```python
from build123d import *

# Parameters (mm, degrees)
F1_DEPTH = 10
F2_R     = 2


# Not quite as in the source:
# - ends of sketch curves that miss each other by under 0.0002 mm in the source are joined


with BuildPart() as f1:
    # F0 (on Front) → F1 (new body)
    with BuildSketch(Plane.XZ):
        Polygon((-0.0010415313, 0.600002712), (-2.25, 0.6039066758), (-2.25, 10), (-5.25, 10), (-5.25, 3), (-10, 3), (-10, 0), (0, 0), align=None)
        Polygon((0.0010415376, 0.599999096), (-0.0010415313, 0.600002712), (0, 0), align=None)
        Polygon((2.25, 0.6039066758), (0.0010415313, 0.600002712), (0, 0), (10, 0), (10, 3), (5.25, 3), (5.25, 10), (2.25, 10), align=None)
    extrude(amount=F1_DEPTH)

    # F2
    f2_edges = [f1.edges().sort_by_distance(p)[0] for p in [
        (-5.25, -5, 3),
        (5.25, -5, 3),
        (10, -5, 3),
        (5.25, -5, 10),
        (-5.25, -5, 10),
        (-10, -5, 3),
        (-10, -10, 1.5),
        (-10, 0, 1.5),
        (10, -10, 1.5),
        (10, 0, 1.5),
    ]]
    fillet(f2_edges, radius=F2_R)


solid = f1.part
```
Part model, mm, in its own coordinate system. A direction names the side the tool comes from. Round coordinates to 2 decimals unless told otherwise and drop trailing zeros. Write each loop counter-clockwise with the first axis right and the second up, starting at its lowest first coordinate (ties: lowest second). Pieces come first, ordered by that corner, then holes. Notation, with made-up numbers: M 40.25,-27 L 81.25,-27 A36 ccw 81.25,11 Z; hole C 39,18.25 d4. An arc over 180 degrees is marked long. One line per question, with ' | ' between items.
(1) Pin check, flat tips, straight feed: pin 1 (0.6 mm diameter, centred on x = 8, y = -3.5, fed in from +Z); pin 2 (2.5 mm diameter, centred on y = -2.5, z = 6.5, fed in from +X); pin 3 (2.5 mm diameter, centred on y = -4.5, z = 7, fed in from -X). Stop position of each tip, or through.
Answer key:
pin 1: stops at z = 3 | pin 2: stops at x = 5.25 | pin 3: stops at x = -5.25
(2) Saw through at D-D on x = -7.5. Write the cut outline in (y, z).
Answer key:
outline: M -10,0 L 0,0 L 0,3 L -10,3 Z
(3) 3-axis set-ups, long thin cutter, end or side, ignore diameter. For faces 1 (the face through (5.85, -5.07, 3.57)), 2 (the face through (2.25, -5, 5)): which of +Z, -Z, +X, -X, +Y, -Y reach the whole face in a straight line?
Answer key:
face 1: +Z, +X, +Y, -Y | face 2: +Z, +Y, -Y
(4) Probe line 1 along X through (y, z) = (-6, 6); line 2 along X through (y, z) = (-5, 4.5); line 3 along Z through (x, y) = (-1.75, -8). List the from-to ranges inside material, lowest first.
Answer key:
line 1: x = -5.25 to -2.25, 2.25 to 5.25 | line 2: x = -5.31 to -2.25, 2.25 to 5.31 | line 3: z = 0 to 0.6
(5) Two-plate mould, pull along X, no slides. Class faces 3 (the face through (-10, -5, 0.5)), 4 (the face through (5.25, -5, 6)), 5 (the face through (-2.25, -5, 5)): released by +X, released by -X, zero draft, split by the parting line, or undercut.
Answer key:
face 3: released by -X | face 4: released by +X | face 5: undercut
(6) Saw through at C-C on z = 2.5. Write the cut outline in (x, y).
Answer key:
outline: M -9.32,-9.5 A2 ccw -8,-10 L -2.25,-10 L -2.25,0 L -8,0 A2 ccw -9.32,-0.5 Z; M 2.25,-10 L 8,-10 A2 ccw 9.32,-9.5 L 9.32,-0.5 A2 ccw 8,0 L 2.25,0 Z
(7) Saw through at A-A on z = 6. Write the cut outline in (x, y).
Answer key:
outline: M -5.25,-10 L -2.25,-10 L -2.25,0 L -5.25,0 Z; M 2.25,-10 L 5.25,-10 L 5.25,0 L 2.25,0 Z
